```python
from build123d import *

# Parameters (mm, degrees)
RESSALTO_EXTRUS_O2_DEPTH             = 33.5
ESCAREADO_PARA_SFHCS_M31_D           = 3.4
ESCAREADO_PARA_SFHCS_M31_CSINK_D     = 6.72
ESCAREADO_PARA_SFHCS_M31_CSINK_ANGLE = 90
ESBO_O7_R                            = 4
CORTE_EXTRUS_O1_DEPTH                = 125.306073866
CORTE_EXTRUS_O2_DEPTH                = 125.306073866


with BuildPart() as part:
    # Esboço3 → Ressalto-extrusão2 (new body)
    with BuildSketch(Plane(origin=(0, 0, 0), x_dir=(1, 0, 0), z_dir=(0, 1, 0))):
        with BuildLine():
            Line((-21.5, 83.269141943), (-21.5, -9.730858057))
            Line((-21.5, -9.730858057), (21.5, -9.730858057))
            Line((21.5, -9.730858057), (21.5, 83.269141943))
            ThreePointArc((21.5, 83.269141943), (38.688656502, 76.806170703), (54.113307426, 66.841229488))
            Line((54.113307426, 66.841229488), (66.841229488, 54.113307426))
            ThreePointArc((66.841229488, 54.113307426), (86, 0), (66.841229488, -54.113307426))
            Line((66.841229488, -54.113307426), (54.113307426, -66.841229488))
            ThreePointArc((54.113307426, -66.841229488), (45.453875584, -73.006473647), (36.1, -78.056325817))
            Line((36.1, -78.056325817), (-36.1, -78.056325817))
            ThreePointArc((-36.1, -78.056325817), (-45.453875584, -73.006473647), (-54.113307426, -66.841229488))
            Line((-54.113307426, -66.841229488), (-66.841229488, -54.113307426))
            ThreePointArc((-66.841229488, -54.113307426), (-86, 0), (-66.841229488, 54.113307426))
            Line((-66.841229488, 54.113307426), (-54.113307426, 66.841229488))
            ThreePointArc((-54.113307426, 66.841229488), (-38.688656502, 76.806170703), (-21.5, 83.269141943))
        make_face()
    extrude(amount=RESSALTO_EXTRUS_O2_DEPTH)

    # Escareado para SFHCS M31 (through all)
    with Locations(Plane(origin=(0, 33.5, 0), x_dir=(1, 0, 0), z_dir=(0, 1, 0))):
        with Locations((45.886114908, 65.532163543), (65.532163543, -45.886114908), (-65.532163543, -45.886114908), (-45.886114908, 65.532163543)):
            CounterSinkHole(ESCAREADO_PARA_SFHCS_M31_D / 2, ESCAREADO_PARA_SFHCS_M31_CSINK_D / 2, counter_sink_angle=ESCAREADO_PARA_SFHCS_M31_CSINK_ANGLE)

    # Esboço7 → Corte-extrusão1 (cut, through all)
    with BuildSketch(Plane(origin=(0, 33.5, 0), x_dir=(1, 0, 0), z_dir=(0, 1, 0))):
        with Locations(Location((-27.361611466, 75.175409663, 0), (0, 0, 270))):
            Circle(ESBO_O7_R)
        with Locations(Location((-47.022820183, -64.72135955, 0), (0, 0, 270))):
            Circle(ESBO_O7_R)
        with Locations(Location((47.022820183, -64.72135955, 0), (0, 0, 90))):
            Circle(ESBO_O7_R)
        with Locations(Location((27.361611466, 75.175409663, 0), (0, 0, 90))):
            Circle(ESBO_O7_R)
    extrude(amount=-CORTE_EXTRUS_O1_DEPTH, mode=Mode.SUBTRACT)

    # Esboço9 → Corte-extrusão2 (cut, through all)
    with BuildSketch(Plane(origin=(0, 33.5, 0), x_dir=(1, 0, 0), z_dir=(0, 1, 0))):
        Polygon((-66.841229488, -54.113307426), (-54.113307426, -66.841229488), (-51.284880301, -64.012802363), (-64.012802363, -51.284880301), align=None)
        Polygon((51.284880301, -64.012802363), (64.012802363, -51.284880301), (66.841229488, -54.113307426), (54.113307426, -66.841229488), align=None)
        Polygon((54.113307426, 66.841229488), (51.284880301, 64.012802363), (64.012802363, 51.284880301), (66.841229488, 54.113307426), align=None)
        Polygon((-51.284880301, 64.012802363), (-64.012802363, 51.284880301), (-66.841229488, 54.113307426), (-54.113307426, 66.841229488), align=None)
    extrude(amount=-CORTE_EXTRUS_O2_DEPTH, mode=Mode.SUBTRACT)


solid = part.part
```
Build history of the part. All positions in model axes, mm. A direction names the side the tool comes from. Round coordinates to 2 decimals unless told otherwise and drop trailing zeros. Loops run counter-clockwise (first coordinate to the right, second up) from the corner with the lowest first, then second, coordinate; pieces in that order, holes last. Notation, with made-up numbers: M -6,84.5 L 51,84.5 A27 ccw 51,118.5 Z; hole C 28,44.25 d4. An arc over 180 degrees is marked long. Answer as CSV lines item,"result".
1. Cut at C-C on y = 17. Count the separate pieces of the cut face and the enclosed holes in it, then the cut area to 3 significant figures.
Resolved:
separate pieces,"1"
enclosed holes,"8"
area,"18,200 mm²"
2. Flat gauge pins, fed straight in: P1, Ø10, axis at x = -6.5, y = 13.5, coming from the -Z side; P2, Ø10, axis at y = 16.5, z = -19.5, coming from the -X side; P3, Ø4, axis at x = -62, y = 26, coming from the -Z side. Where does each tip first touch, or does it go through?
Resolved:
P1,"stops at z = 9.73"
P2,"stops at x = -84.77"
P3,"stops at z = -55.3"
3. 3-axis set-ups, long thin cutter, end or side, ignore diameter. For faces 4 (the flat face through (-21.5, 17, -37)), 5 (the cylindrical face through (-45.3, 16.5, 73.1)), 6 (the flat face through (57.6, 17, -57.7)): which of +Z, -Z, +X, -X, +Y, -Y reach the whole face in a straight line?
Resolved:
face 4,"-Z, +Y, -Y"
face 5,"+Z, -X, +Y, -Y"
face 6,"+Y, -Y"
4. Cut at B-B on x = -17. Write the cut outline in (y, z), then the cut area to 3 significant figures.
Resolved:
outline,"M 0,9.73 L 33.5,9.73 L 33.5,78.06 L 0,78.06 Z"
area,"2,290 mm²"
5. Two-plate mould, pull along X, no slides. Class faces 1 (the cylindrical face through (38.5, 16.5, -76.9)), 2 (the flat face through (57.6, 17, 57.7)), 3 (the flat face through (1, 17, 78.056)): released by +X, released by -X, zero draft, split by the parting line, or undercut.
Resolved:
face 1,"released by +X"
face 2,"undercut"
face 3,"zero draft"
6. Cut at D-D on z = 6. Write the cut outline in (x, y).
Resolved:
outline,"M -85.79,0 L -21.5,0 L -21.5,33.5 L -85.79,33.5 Z; M 21.5,0 L 85.79,0 L 85.79,33.5 L 21.5,33.5 Z"
7. Wall check: probe 1 along X at (y, z) = (11, 64); probe 2 along Z at (x, y) = (45.5, 26); probe 3 along X at (y, z) = (25, -2). Give the ranges that are in metal, low to high. Write a range as [from, to].
Resolved:
probe 1,"x = [-51.3, -50.96], [-43.09, 43.09], [50.96, 51.3]"
probe 2,"z = [-72.98, -67.19], [-63.88, 61.02], [68.42, 72.98]"
probe 3,"x = [-85.98, -21.5], [21.5, 85.98]"
8. Cut at A-A on z = -44.5. Write the cut outline in (x, y), then the cut area to 3 significant figures.
Resolved:
outline,"M -73.59,0 L -21.5,0 L -21.5,33.5 L -73.59,33.5 Z; M 21.5,0 L 73.59,0 L 73.59,33.5 L 21.5,33.5 Z"
area,"3,490 mm²"
